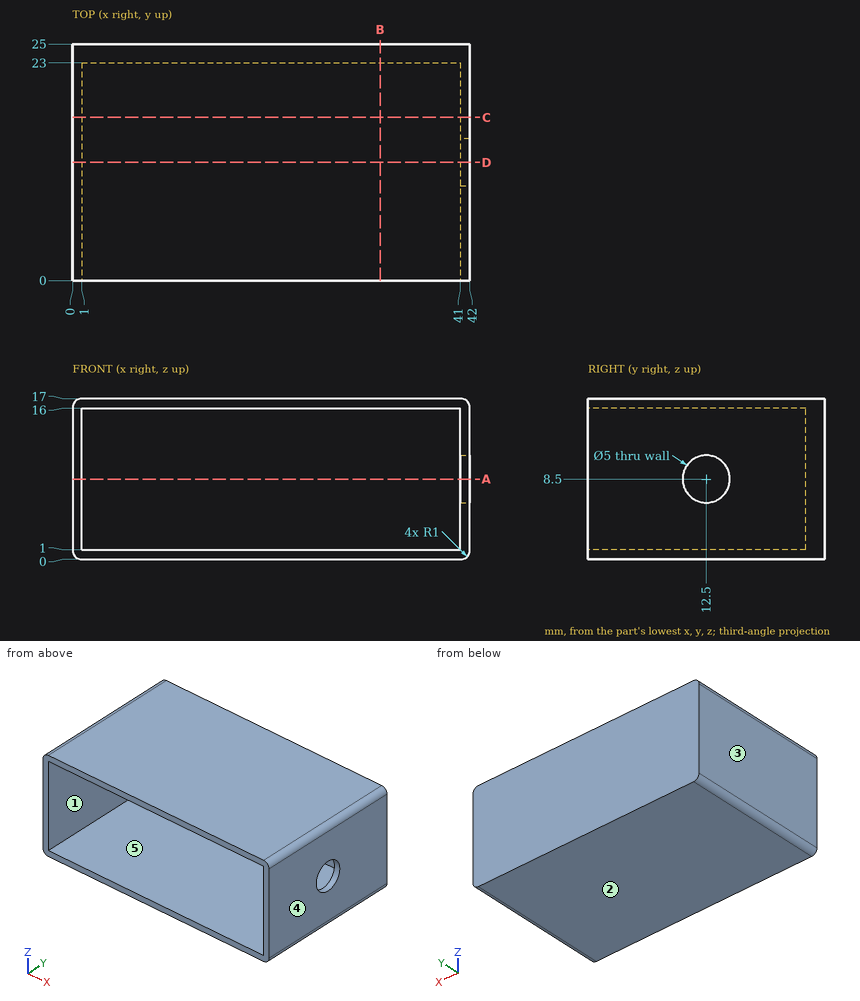
Verification items for this drawing (mm, ordinates from the low corner). A direction names the side the tool comes from. Coordinates: 2 decimals unless noted, no trailing zeros. Write each loop counter-clockwise with the first axis right and the second up, starting at its lowest first coordinate (ties: lowest second). Pieces come first, ordered by that corner, then holes. Notation, with made-up numbers: M 45.5,4.5 L 57.5,4.5 A23 ccw 57.5,26.5 Z; hole C -18.75,89.5 d4. An arc over 180 degrees is marked long. Answer as CSV lines item,"result".
Q1. Cross-section at B-B (x = 32.5). Record the boundary of the cut face in (y, z), then the cut area to 3 significant figures.
Check result:
outline,"M 0,0 L 25,0 L 25,17 L 0,17 L 0,16 L 23,16 L 23,1 L 0,1 Z"
area,"80.0 mm^2"
Q2. Mould release check, pull along X, two halves, no side actions. Record for the marked faces 3, 4 and 5: released by +X, released by -X, zero draft, split by the parting line, or undercut.
Check result:
face 3,"released by -X"
face 4,"released by +X"
face 5,"undercut"
Q3. Cross-section at D-D (y = 12.5). Record the boundary of the cut face in (x, z).
Check result:
outline,"M 0,1 A1 ccw 1,0 L 41,0 A1 ccw 42,1 L 42,6 L 41,6 L 41,1 L 1,1 L 1,16 L 41,16 L 41,11 L 42,11 L 42,16 A1 ccw 41,17 L 1,17 A1 ccw 0,16 Z"
Q4. Go/stop test with flat-tipped pins: pin 1 (4 mm diameter, centred on y = 11.5, z = 7.5, fed in from +X); pin 2 (7.5 mm diameter, centred on x = 25, z = 11.5, fed in from -Y). Record where each tip stops, or that it passes through.
Check result:
pin 1,"x = 42"
pin 2,"y = 23"
Q5. Material ranges on probe 1 along X at (y, z) = (9.5, 10.5); probe 2 along Z at (x, y) = (9, 7.75); probe 3 along Z at (x, y) = (41.55, 12.5), recorded low to high. Write a range as from..to.
Check result:
probe 1,"0..1, 41..42"
probe 2,"0..1, 16..17"
probe 3,"0.16..6, 11..16.84"
Q6. Cross-section at C-C (y = 17.25). Record the boundary of the cut face in (x, z).
Check result:
outline,"M 0,1 A1 ccw 1,0 L 41,0 A1 ccw 42,1 L 42,16 A1 ccw 41,17 L 1,17 A1 ccw 0,16 Z; hole M 1,1 L 41,1 L 41,16 L 1,16 Z"
Q7. Cross-section at A-A (z = 8.5). Record the boundary of the cut face in (x, y), then the cut area to 3 significant figures.
Check result:
outline,"M 0,0 L 1,0 L 1,23 L 41,23 L 41,15 L 42,15 L 42,25 L 0,25 Z; M 41,0 L 42,0 L 42,10 L 41,10 Z"
area,"125 mm^2"
Q8. Set-up check for the marked faces 1 and 2: record each of +Z, -Z, +X, -X, +Y, -Y from which the full face is reachable in a straight line by a thin tool's end or side.
Check result:
face 1,"-Y"
face 2,"-Z, +X, -X, +Y, -Y"
